```python
from build123d import *

# Parameters (mm, degrees)
BOSS_EXTRUDE1_DEPTH = 5
SKETCH3_W           = 5
SKETCH3_H           = 30
BOSS_EXTRUDE3_DEPTH = 22
BOSS_EXTRUDE4_DEPTH = 5
SKETCH5_R           = 1.5
SKETCH5_R_2         = 2
CUT_EXTRUDE1_DEPTH  = 29.166222313
FILLET1_R           = 4
CUT_EXTRUDE2_START  = -1
CUT_EXTRUDE2_DEPTH  = 24
CUT_EXTRUDE3_DEPTH  = 2.3


with BuildPart() as part:
    # Sketch2 → Boss-Extrude1 (new body)
    with BuildSketch(Plane(origin=(0, 0, 0), x_dir=(1, 0, 0), z_dir=(0, 1, 0))):
        with BuildLine():
            Line((18, -15), (18, 15))
            Line((18, 15), (0, 15))
            ThreePointArc((0, 15), (-5.457051563, 13.972136137), (-10.166222313, 11.029411765))
            Line((-10.166222313, 11.029411765), (-5.760859311, 6.25))
            ThreePointArc((-5.760859311, 6.25), (8.5, 0), (-5.760859311, -6.25))
            Line((-5.760859311, -6.25), (-10.166222313, -11.029411765))
            ThreePointArc((-10.166222313, -11.029411765), (-5.457051563, -13.972136137), (0, -15))
            Line((0, -15), (18, -15))
        make_face()
    extrude(amount=BOSS_EXTRUDE1_DEPTH)

    # Sketch3 → Boss-Extrude3 (add)
    with BuildSketch(Plane(origin=(0, 5, 0), x_dir=(1, 0, 0), z_dir=(0, 1, 0))):
        with Locations((15.5, 0)):
            Rectangle(SKETCH3_W, SKETCH3_H)
    extrude(amount=BOSS_EXTRUDE3_DEPTH)

    # Sketch4 → Boss-Extrude4 (add)
    with BuildSketch(Plane(origin=(0, 27, 0), x_dir=(1, 0, 0), z_dir=(0, 1, 0))):
        with BuildLine():
            Line((13, -15), (18, -15))
            Line((18, -15), (18, 15))
            Line((18, 15), (13, 15))
            Line((13, 15), (0, 15))
            ThreePointArc((0, 15), (-5.457051563, 13.972136137), (-10.166222313, 11.029411765))
            Line((-10.166222313, 11.029411765), (-5.760859311, 6.25))
            ThreePointArc((-5.760859311, 6.25), (8.5, 0), (-5.760859311, -6.25))
            Line((-5.760859311, -6.25), (-10.166222313, -11.029411765))
            ThreePointArc((-10.166222313, -11.029411765), (-5.457051563, -13.972136137), (0, -15))
            Line((0, -15), (13, -15))
        make_face()
    extrude(amount=BOSS_EXTRUDE4_DEPTH)

    # Sketch5 → Cut-Extrude1 (cut, through all)
    with BuildSketch(Plane(origin=(18, 0, 0), x_dir=(0, 0, -1), z_dir=(1, 0, 0))):
        with Locations((9, 23)):
            Circle(SKETCH5_R)
        with Locations((-9, 9)):
            Circle(SKETCH5_R)
        with Locations((-9, 23)):
            Circle(SKETCH5_R_2)
        with Locations((9, 9)):
            Circle(SKETCH5_R_2)
    extrude(amount=-CUT_EXTRUDE1_DEPTH, mode=Mode.SUBTRACT)

    # Fillet1
    fillet1_edges = [part.edges().sort_by_distance(p)[0] for p in [
        (-10.166222313, 2.5, 11.029411765),
        (-10.166222313, 2.5, -11.029411765),
        (-10.166222313, 29.5, 11.029411765),
        (-10.166222313, 29.5, -11.029411765),
    ]]
    fillet(fillet1_edges, radius=FILLET1_R)

    # Sketch6 → Cut-Extrude2 (cut)
    with BuildSketch(Plane.XZ.offset(-27).offset(CUT_EXTRUDE2_START)):
        with BuildLine():
            Line((-7.951245646, -9.6), (0, -9.6))
            ThreePointArc((0, -9.6), (-3.492513001, -8.942167128), (-6.506382281, -7.058823529))
            Line((-6.506382281, -7.058823529), (-6.944851968, -7.534522622))
            ThreePointArc((-6.944851968, -7.534522622), (-7.59954211, -8.493446945), (-7.951245646, -9.6))
        make_face()
        with BuildLine():
            ThreePointArc((9.6, 0), (6.788225099, 6.788225099), (0, 9.6))
            ThreePointArc((0, 9.6), (-3.492513001, 8.942167128), (-6.506382281, 7.058823529))
            Line((-6.506382281, 7.058823529), (-5.760859311, 6.25))
            ThreePointArc((-5.760859311, 6.25), (8.5, 0), (-5.760859311, -6.25))
            Line((-5.760859311, -6.25), (-6.506382281, -7.058823529))
            ThreePointArc((-6.506382281, -7.058823529), (-3.492513001, -8.942167128), (0, -9.6))
            ThreePointArc((0, -9.6), (6.788225099, -6.788225099), (9.6, 0))
        make_face()
        with BuildLine():
            Line((-5.760859311, 6.25), (-6.506382281, 7.058823529))
            ThreePointArc((-6.506382281, 7.058823529), (-8.792646641, 3.853487389), (-9.6, 0))
            ThreePointArc((-9.6, 0), (-8.792646641, -3.853487389), (-6.506382281, -7.058823529))
            Line((-6.506382281, -7.058823529), (-5.760859311, -6.25))
            ThreePointArc((-5.760859311, -6.25), (8.5, 0), (-5.760859311, 6.25))
        make_face()
        with BuildLine():
            ThreePointArc((-6.506382281, 7.058823529), (-3.492513001, 8.942167128), (0, 9.6))
            Line((0, 9.6), (-7.951245646, 9.6))
            ThreePointArc((-7.951245646, 9.6), (-7.59954211, 8.493446945), (-6.944851968, 7.534522622))
            Line((-6.944851968, 7.534522622), (-6.506382281, 7.058823529))
        make_face()
    extrude(amount=CUT_EXTRUDE2_DEPTH, mode=Mode.SUBTRACT)

    # Sketch7 → Cut-Extrude3 (cut)
    with BuildSketch(Plane.ZY.offset(-13)):
        Polygon((-4.958548116, 9), (-6.979274058, 12.5), (-11.020725942, 12.5), (-13.041451884, 9), (-11.020725942, 5.5), (-6.979274058, 5.5), align=None)
        Polygon((13.041451884, 23), (11.020725942, 26.5), (6.979274058, 26.5), (4.958548116, 23), (6.979274058, 19.5), (11.020725942, 19.5), align=None)
    extrude(amount=-CUT_EXTRUDE3_DEPTH, mode=Mode.SUBTRACT)


solid = part.part
```
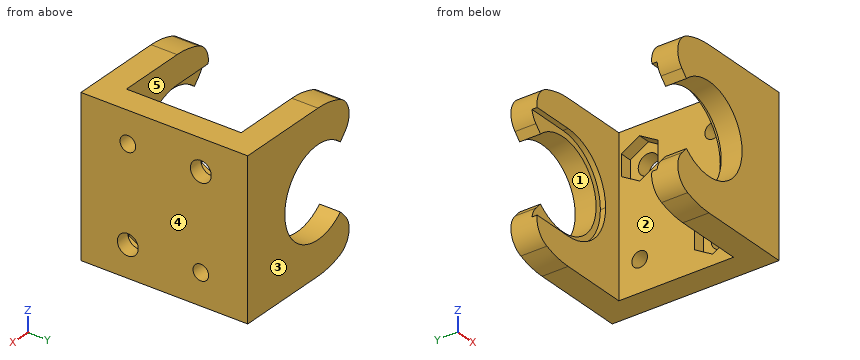
Geometry check sheet. Reference: the model listing, model coordinates, mm. Face numbers are marked on the shaded views. A direction names the side the tool comes from. Coordinates: 2 decimals unless noted, no trailing zeros. Order: outer loops, then holes, each group sorted by start corner. A loop starts at its lowest first (then second) coordinate and runs counter-clockwise, first axis right, second up.
Item 1: Mould release check, pull along Y, two halves, no side actions. Record for the marked faces 3, 4 and 5: released by +Y, released by -Y, zero draft, split by the parting line, or undercut.
Item 2: Scan lines: line 1 along Y through (x, z) = (17.1, -9); line 2 along Y through (x, z) = (16.7, 9); line 3 along Y through (x, z) = (7.5, -6.25). Record each from-to range of solid material in increasing order.
Item 3: Section check D-D (y = 9.5). Enter the section's corners in (x, z), plus the area to 3 significant figures.
Item 4: Section check A-A (z = -9). Enter the section's corners in (x, y), plus the area to 3 significant figures.
Item 5: Section check C-C (x = -3.75). Enter the section's corners in (y, z).
Item 6: Depth check by flat-ended pin: pin 1 (0.5 mm diameter, centred on x = -5, y = 4.5, fed in from +Z); pin 2 (4 mm diameter, centred on y = 9, z = 9, fed in from -X); pin 3 (5 mm diameter, centred on y = 23, z = -9, fed in from +X); pin 4 (0.8 mm diameter, centred on x = -3, y = 27.5, fed in from -Z). Enter the tip coordinate at first touch or a pass-through.
Item 7: Section check B-B (x = 13.75). Enter the section's corners in (y, z), plus the area to 3 significant figures.
Item 8: Tool access check on the marked faces 1 and 2. Record the directions out of +Z, -Z, +X, -X, +Y, -Y that give a thin tool (end or side, any length) a straight path to the whole face; none if there is none.
Check sheet entries:
1. face 3: released by +Y
1. face 4: zero draft
1. face 5: undercut
2. line 1: y = 0 to 7, 11 to 21.5, 24.5 to 32
2. line 2: y = 0 to 7.5, 10.5 to 21, 25 to 32
2. line 3: y = 0 to 5, 27 to 32
3. outline: (13, -15) - (18, -15) - (18, -10.94) - (15.3, -10.94) - (15.3, -12.75) - (13, -12.75) - close; (13, -5.25) - (15.3, -5.25) - (15.3, -7.06) - (18, -7.06) - (18, 7.59) - (13, 7.59) - close; (13, 10.41) - (18, 10.41) - (18, 15) - (13, 15) - close
3. area: 108 mm2
4. outline: (-7.8, 0) - (18, 0) - (18, 7) - (15.3, 7) - (15.3, 5.5) - (13, 5.5) - (13, 5) - (3.34, 5) - (3.34, 4) - (-7.8, 4) - close; (-7.8, 28) - (3.34, 28) - (3.34, 27) - (13, 27) - (13, 24.5) - (18, 24.5) - (18, 32) - (-7.8, 32) - close; (13, 12.5) - (15.3, 12.5) - (15.3, 11) - (18, 11) - (18, 21.5) - (13, 21.5) - close
4. area: 304 mm2
5. outline: (0, -14.52) - (5, -14.52) - (5, -9.6) - (4, -9.6) - (4, -7.63) - (0, -7.63) - close; (0, 7.63) - (4, 7.63) - (4, 9.6) - (5, 9.6) - (5, 14.52) - (0, 14.52) - close; (27, -14.52) - (32, -14.52) - (32, -7.63) - (28, -7.63) - (28, -9.6) - (27, -9.6) - close; (27, 9.6) - (28, 9.6) - (28, 7.63) - (32, 7.63) - (32, 14.52) - (27, 14.52) - close
6. pin 1: stops at z = 14.23
6. pin 2: stops at x = 13
6. pin 3: stops at x = 18
6. pin 4: stops at z = -14.77
7. outline: (0, -15) - (32, -15) - (32, 15) - (0, 15) - close; hole (5.5, -11.02) - (9, -13.04) - (12.5, -11.02) - (12.5, -6.98) - (9, -4.96) - (5.5, -6.98) - close; hole circle Ø3 at (9, 9); hole (19.5, 6.98) - (23, 4.96) - (26.5, 6.98) - (26.5, 11.02) - (23, 13.04) - (19.5, 11.02) - close; hole circle Ø3 at (23, -9)
7. area: 861 mm2
8. face 1: +Y, -Y
8. face 2: +Z, -Z, -X
